```python
from build123d import *

# Parameters (mm, degrees)
F0_R     = 12.5
F1_DEPTH = 12


with BuildPart() as f1:
    # F0 (on Front) → F1 (new body)
    with BuildSketch(Plane.XZ):
        with BuildLine():
            ThreePointArc((176.1118317896, -31.230215018), (197.4867432438, -21.7004349792), (206.25, 0))
            ThreePointArc((206.25, 0), (197.4867432438, 21.7004349792), (176.1118317896, 31.230215018))
            ThreePointArc((176.1118317896, 31.230215018), (143.75, 0), (176.1118317896, -31.230215018))
        make_face()
        with Locations((175, 0)):
            Circle(F0_R, mode=Mode.SUBTRACT)
        with BuildLine():
            ThreePointArc((176.1118317896, -31.230215018), (143.75, 0), (176.1118317896, 31.230215018))
            Line((176.1118317896, 31.230215018), (72.8595976104, 34.9061140228))
            ThreePointArc((72.8595976104, 34.9061140228), (51.3833504258, 45.0935396139), (44.0597993868, 67.7072176317))
            Line((44.0597993868, 67.7072176317), (59.4515870825, 230.7189524824))
            ThreePointArc((59.4515870825, 230.7189524824), (0, 187.5), (-59.4515870825, 230.7189524824))
            Line((-59.4515870825, 230.7189524824), (-37.3339459271, -3.5251214894))
            ThreePointArc((-37.3339459271, -3.5251214894), (-1.7645151934, 37.458463478), (37.5, 0))
            ThreePointArc((37.5, 0), (27.4431367381, -25.556295623), (2.6667068815, -37.4050621495))
            Line((2.6667068815, -37.4050621495), (176.1118317896, -31.230215018))
        make_face()
        with BuildLine():
            Line((0, -37.5), (2.6667068815, -37.4050621495))
            ThreePointArc((2.6667068815, -37.4050621495), (27.4431367381, -25.556295623), (37.5, 0))
            ThreePointArc((37.5, 0), (-1.7645151934, 37.458463478), (-37.3339459271, -3.5251214894))
            ThreePointArc((-37.3339459271, -3.5251214894), (-25.2394328794, -27.7348341969), (0, -37.5))
        make_face()
        Circle(F0_R, mode=Mode.SUBTRACT)
        with BuildLine():
            ThreePointArc((0, -37.5), (1.3341981475, -37.4762580216), (2.6667068815, -37.4050621495))
            Line((2.6667068815, -37.4050621495), (0, -37.5))
        make_face()
        with BuildLine():
            Line((62.0097963531, 257.8125), (59.4515870825, 230.7189524824))
            ThreePointArc((59.4515870825, 230.7189524824), (61.7331928247, 240.2397282992), (62.5, 250))
            ThreePointArc((62.5, 250), (62.3773287023, 253.9139320339), (62.0097963531, 257.8125))
        make_face()
        with BuildLine():
            ThreePointArc((-59.4515870825, 230.7189524824), (0, 187.5), (59.4515870825, 230.7189524824))
            Line((59.4515870825, 230.7189524824), (62.0097963531, 257.8125))
            ThreePointArc((62.0097963531, 257.8125), (0, 312.5), (-62.0097963531, 257.8125))
            Line((-62.0097963531, 257.8125), (-59.4515870825, 230.7189524824))
        make_face()
        with Locations((0, 250)):
            Circle(F0_R, mode=Mode.SUBTRACT)
        with BuildLine():
            ThreePointArc((-62.0097963531, 257.8125), (-62.2232432118, 244.1247975176), (-59.4515870825, 230.7189524824))
            Line((-59.4515870825, 230.7189524824), (-62.0097963531, 257.8125))
        make_face()
        with BuildLine():
            ThreePointArc((-62.0097963531, 257.8125), (0, 312.5), (62.0097963531, 257.8125))
            Line((62.0097963531, 257.8125), (37.2058778118, 454.6875))
            ThreePointArc((37.2058778118, 454.6875), (37.4263972214, 452.3483592204), (37.5, 450))
            ThreePointArc((37.5, 450), (-2.3483592204, 412.5736027786), (-37.2058778118, 454.6875))
            Line((-37.2058778118, 454.6875), (-62.0097963531, 257.8125))
        make_face()
        with Locations((-12.5, 394)):
            Circle(F0_R, mode=Mode.SUBTRACT)
        with BuildLine():
            ThreePointArc((37.5, 450), (37.4263972214, 452.3483592204), (37.2058778118, 454.6875))
            ThreePointArc((37.2058778118, 454.6875), (0, 487.5), (-37.2058778118, 454.6875))
            ThreePointArc((-37.2058778118, 454.6875), (-2.3483592204, 412.5736027786), (37.5, 450))
        make_face()
        with Locations((0, 450)):
            Circle(F0_R, mode=Mode.SUBTRACT)
    extrude(amount=F1_DEPTH)


solid = f1.part
```
Geometry check sheet. Reference: the model listing, model coordinates, mm. A direction names the side the tool comes from. Coordinates: 2 decimals unless noted, no trailing zeros. Loops run counter-clockwise (first coordinate to the right, second up) from the corner with the lowest first, then second, coordinate; pieces in that order, holes last. Notation, with made-up numbers: (76.5, -21) - (113.5, -21) arc R18 ccw to (113.5, -4) - close; hole circle Ø2 at (85, -31). An arc over 180 degrees is marked (long way). One line per item, written item: value. Start each with the question number.
(1) Material ranges on line 1 (Z direction, x = 4.5, y = -3); line 2 (Z direction, x = -15, y = -9.75); line 3 (X direction, y = -9.75, z = 401.5), recorded low to high. Write a range as [from, to].
(2) Tool access check on faces 5 (the flat face through (10, -12, 170)), 6 (the flat face through (51.648, -5.916, 148.072)). Record the directions out of +Z, -Z, +X, -X, +Y, -Y that give a thin tool (end or side, any length) a straight path to the whole face; none if there is none.
(3) Depth check by flat-ended pin: P1, Ø6, axis at x = -20.5, z = 165.5, coming from the +Y side; P2, Ø1.5, axis at x = 35, y = -2, coming from the +Z side; P3, Ø4, axis at x = 86, y = -5, coming from the -Z side; P4, Ø6, axis at y = -9.5, z = 277.5, coming from the +X side. Enter the tip coordinate at first touch or a pass-through.
(4) Cross-section at C-C on z = 394. Enter the section's corners in (x, y).
(5) Cross-section at A-A on y = -9.75. Enter the section's corners in (x, z), plus the area to 3 significant figures.
(6) Cross-section at B-B on x = -18. Enter the section's corners in (y, z), plus the area to 3 significant figures.
(7) Mould release check, pull along X, two halves, no side actions. Record for faces 1 (the cylindrical face through (-62.24, -5.92, 244.32)), 2 (the cylindrical face through (51.61, -5.92, 44.84)), 3 (the cylindrical face through (5.77, -5.92, 438.91)), 4 (the cylindrical face through (0.759, -5.916, 487.492)): released by +X, released by -X, zero draft, split by the parting line, or undercut.
(8) Cross-section at D-D on z = 121. Enter the section's corners in (x, y).
Results below:
1. line 1: z = [-37.34, -11.66], [11.66, 238.34], [261.66, 438.34], [461.66, 487.23]
1. line 2: z = [-34.37, 381.75], [406.25, 484.37]
1. line 3: x = [-43.91, -22.5], [-2.5, 43.91]
2. face 5: +Z, -Z, +X, -X, -Y
2. face 6: +X, +Y, -Y
3. P1: stops at y = 0
3. P2: stops at z = 465.27
3. P3: stops at z = -34.51
3. P4: stops at x = 59.91
4. outline: (-44.85, -12) - (-25, -12) - (-25, 0) - (-44.85, 0) - close; (0, -12) - (44.85, -12) - (44.85, 0) - (0, 0) - close
5. outline: (-62.01, 257.81) arc R62.5 ccw to (-59.45, 230.72) - (-37.33, -3.53) arc R37.5 ccw to (2.67, -37.41) - (176.11, -31.23) arc R31.25 ccw to (176.11, 31.23) - (72.86, 34.91) arc R30 cw to (44.06, 67.71) - (59.45, 230.72) arc R62.5 ccw to (62.01, 257.81) - (37.21, 454.69) arc R37.5 ccw to (-37.21, 454.69) - close; hole circle Ø25 at (-12.5, 394); hole circle Ø25 at (0, 0); hole circle Ø25 at (0, 250); hole circle Ø25 at (0, 450); hole circle Ø25 at (175, 0)
5. area: 58,100 mm2
6. outline: (-12, -32.9) - (0, -32.9) - (0, 382.78) - (-12, 382.78) - close; (-12, 405.22) - (0, 405.22) - (0, 482.9) - (-12, 482.9) - close
6. area: 5,920 mm2
7. face 1: released by -X
7. face 2: released by +X
7. face 3: undercut
7. face 4: split by the parting line
8. outline: (-49.09, -12) - (49.09, -12) - (49.09, 0) - (-49.09, 0) - close
